```python
from build123d import *

# Parameters (mm, degrees)
F1_DEPTH = 0.5


with BuildPart() as f1:
    # F0 (on Front) → F1 (new body, symmetric)
    with BuildSketch(Plane.XZ):
        with BuildLine():
            Line((-3.5, 0.75), (-3.5, 1.5))
            ThreePointArc((-3.5, 1.5), (-5, 0), (-3.5, -1.5))
            Line((-3.5, -1.5), (-3.5, -0.75))
            ThreePointArc((-3.5, -0.75), (-4.25, 0), (-3.5, 0.75))
        make_face()
        with BuildLine():
            ThreePointArc((3.5, -1.5), (5, 0), (3.5, 1.5))
            Line((3.5, 1.5), (3.5, 0.75))
            ThreePointArc((3.5, 0.75), (4.0303300859, 0.5303300859), (4.25, 0))
            ThreePointArc((4.25, 0), (4.0303300859, -0.5303300859), (3.5, -0.75))
            Line((3.5, -0.75), (3.5, -1.5))
        make_face()
        with BuildLine():
            Line((3.5, 1.5), (-3.5, 1.5))
            Line((-3.5, 1.5), (-3.5, 0.75))
            ThreePointArc((-3.5, 0.75), (-2.9696699141, 0.5303300859), (-2.75, 0))
            ThreePointArc((-2.75, 0), (-2.9696699141, -0.5303300859), (-3.5, -0.75))
            Line((-3.5, -0.75), (-3.5, -1.5))
            Line((-3.5, -1.5), (3.5, -1.5))
            Line((3.5, -1.5), (3.5, -0.75))
            ThreePointArc((3.5, -0.75), (2.75, 0), (3.5, 0.75))
            Line((3.5, 0.75), (3.5, 1.5))
        make_face()
    extrude(amount=F1_DEPTH, both=True)


solid = f1.part
```
CAD build for the part. Positions are in the model's coordinates, mm. Round coordinates to 2 decimals unless told otherwise and drop trailing zeros. Loops run counter-clockwise (first coordinate to the right, second up) from the corner with the lowest first, then second, coordinate; pieces in that order, holes last. Notation, with made-up numbers: M 45.5,80 L 84.5,80 A20 cw 84.5,116 Z; hole C 10.25,63.5 d3. An arc over 180 degrees is marked long. Return JSON: item names as keys, results as strings. Group by question number.
(1) Saw through at A-A, the plane y = -0.15. List the corners of the cut face in (x, z), and give its area (3 significant figures).
(2) Saw through at B-B, the plane z = 0.4. List the corners of the cut face in (x, y).
(3) Wall check: probe 1 along X at (y, z) = (0.25, 0.05); probe 2 along X at (y, z) = (-0.3, 0.65); probe 3 along Z at (x, y) = (-3.25, 0.2). Give the ranges that are in metal, low to high. Write a range as [from, to].
(4) Saw through at C-C, the plane z = -0.95. List the corners of the cut face in (x, y).
Answer list:
{
 "1": {"outline": "M -3.5,-1.5 L 3.5,-1.5 A1.5 ccw 3.5,1.5 L -3.5,1.5 A1.5 ccw Z; hole C -3.5,0 d1.5; hole C 3.5,0 d1.5", "area": "24.5 mm2"},
 "2": {"outline": "M -4.95,-0.5 L -4.13,-0.5 L -4.13,0.5 L -4.95,0.5 Z; M -2.87,-0.5 L 2.87,-0.5 L 2.87,0.5 L -2.87,0.5 Z; M 4.13,-0.5 L 4.95,-0.5 L 4.95,0.5 L 4.13,0.5 Z"},
 "3": {"probe 1": "[-5, -4.25], [-2.75, 2.75], [4.25, 5]", "probe 2": "[-4.85, -3.87], [-3.13, 3.13], [3.87, 4.85]", "probe 3": "[-1.5, -0.71], [0.71, 1.5]"},
 "4": {"outline": "M -4.66,-0.5 L 4.66,-0.5 L 4.66,0.5 L -4.66,0.5 Z"}
}
